```python
from build123d import *


with BuildPart() as part:
    # Sketch3 → Revolve3 (revolve)
    with BuildSketch(Plane.XY):
        Polygon((7.440423316, 2.54), (7.440423316, 4.826), (0, 4.826), (0, 0), (9.831510881, 0), (9.831510881, 2.54), align=None)
        with BuildLine():
            ThreePointArc((0, 4.826), (5.484183749, 5.979806298), (10.038536816, 9.2456))
            Line((10.038536816, 9.2456), (10.038536816, 4.826))
            Line((10.038536816, 4.826), (7.440423316, 4.826))
            Line((7.440423316, 4.826), (0, 4.826))
        make_face()
    revolve(axis=Axis((0, 0, 0), (0, 1, 0)))


solid = part.part
```
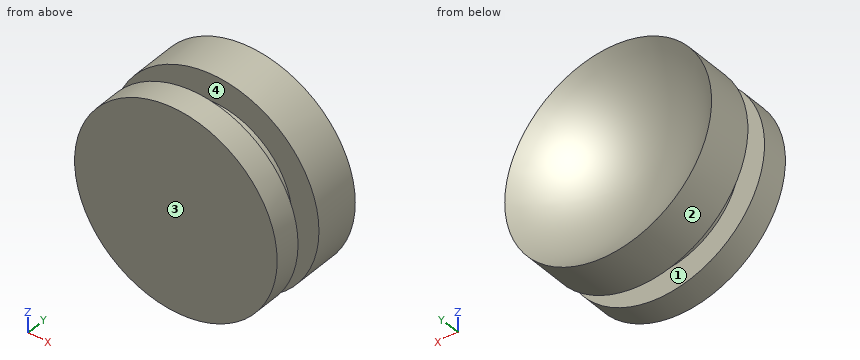
Here's how the part is built. I have some questions about the finished solid (model axes, mm). Face numbers are marked on the shaded views. Coordinates: 2 decimals unless noted, no trailing zeros. Loops run counter-clockwise (first coordinate to the right, second up) from the corner with the lowest first, then second, coordinate; pieces in that order, holes last. Notation, with made-up numbers: (37, 33) - (62, 33) arc R29 cw to (62, 64) - close; hole circle Ø7 at (-36.5, 43). An arc over 180 degrees is marked (long way). Return JSON: item names as keys, results as strings. Group by question number.
Item 1: I need wall thicknesses on line 1 (Y direction, x = 6.5, z = -7); line 2 (X direction, y = 6.25, z = -2.25); line 3 (Y direction, x = -5.5, z = 6). Which ranges of each line are inside material? Lowest first, please. Write a range as from..to.
Item 2: If we section it at C-C on y = 4.5: Write out the boundary of the cut face in (x, z), and give its area (3 significant figures).
Item 3: We'd pull the mould along Y, two halves only. Please class the marked faces 1, 2, 3 and 4: +Y half, -Y half, draft (parallel to the pull), parting line (faces both ways), or undercut.
Item 4: If we section it at A-A on x = 0: Write out the boundary of the cut face in (y, z).
Item 5: If we section it at D-D on y = 6: Write out the boundary of the cut face in (x, z).
Item 6: Will these pins go through, and if not, where does the flat tip stop? P1, Ø2, axis at x = -4.5, z = -2.5, coming from the +Y side; P2, Ø3, axis at y = 8, z = 4, coming from the +X side; P3, Ø10, axis at x = 4, z = -2.5, coming from the +Y side.
Item 7: If we section it at B-B on z = 0: Write out the boundary of the cut face in (x, y).
Calculated:
{
 "1": {"line 1": "y = 0..2.54, 4.83..8.74", "line 2": "x = -9.78..-5.63, 5.63..9.78", "line 3": "y = 0..2.54, 4.83..7.53"},
 "2": {"outline": "circle Ø14.88 at (0, 0)", "area": "174 mm^2"},
 "3": {"face 1": "undercut", "face 2": "draft", "face 3": "-Y half", "face 4": "undercut"},
 "4": {"outline": "(0, -9.83) - (2.54, -9.83) - (2.54, -7.44) - (4.83, -7.44) - (4.83, -10.04) - (9.25, -10.04) arc R13.61 cw to (9.25, 10.04) - (4.83, 10.04) - (4.83, 7.44) - (2.54, 7.44) - (2.54, 9.83) - (0, 9.83) - close"},
 "5": {"outline": "circle Ø20.08 at (0, 0); hole circle Ø11.06 at (0, 0)"},
 "6": {"P1": "stops at y = 6.29", "P2": "stops at x = 9.72", "P3": "stops at y = 8.91"},
 "7": {"outline": "(-10.04, 4.83) - (-7.44, 4.83) - (-7.44, 2.54) - (-9.83, 2.54) - (-9.83, 0) - (9.83, 0) - (9.83, 2.54) - (7.44, 2.54) - (7.44, 4.83) - (10.04, 4.83) - (10.04, 9.25) arc R13.61 cw to (-10.04, 9.25) - close"}
}
